For this review, take the finished solid that the model builds, in its own axes (mm). Face numbers are marked on the shaded views. A direction names the side the tool comes from. Round coordinates to 2 decimals unless told otherwise and drop trailing zeros. Loops run counter-clockwise (first coordinate to the right, second up) from the corner with the lowest first, then second, coordinate; pieces in that order, holes last.
1) Wall thickness on L1, parallel to Z at x = -84, y = -11; L2, parallel to Z at x = -97, y = -3.5; L3, parallel to Z at x = -57.5, y = 8: over which ranges is each line inside the solid? List them lowest first.
2) Take a section at A-A (x = -61). State the section outline as (y, z) points.
3) Take a section at C-C (z = -4). State the section outline as (x, y) points, then the cut area to 3 significant figures.
4) Insertion check: pin 1 (14.5 mm diameter, centred on x = -108.5, z = 19, fed in from +Y); pin 2 (11 mm diameter, centred on x = 27.5, z = -31.5, fed in from -Y); pin 3 (6.5 mm diameter, centred on y = -11, z = 17.06, fed in from +X); pin 4 (3 mm diameter, centred on x = 23.5, z = 16, fed in from -Y). Each pin has a flat end and moves straight along its axis. Give the tip position at first contact, or say it passes through.
5) Mouldability with a two-part tool opening along Z and no side actions: class the marked faces 4, 5 and 6 as pulls with the +Z half, pulls with the -Z half, needs draft (parallel to the pull), parting line crosses it, or undercut.
6) Take a section at B-B (x = 10). State the section outline as (y, z) points.
7) Tool access review of the marked faces 1, 2 and 3: name each direction out of +Z, -Z, +X, -X, +Y, -Y from which nothing blocks a thin tool from reaching the whole face with its end or side.
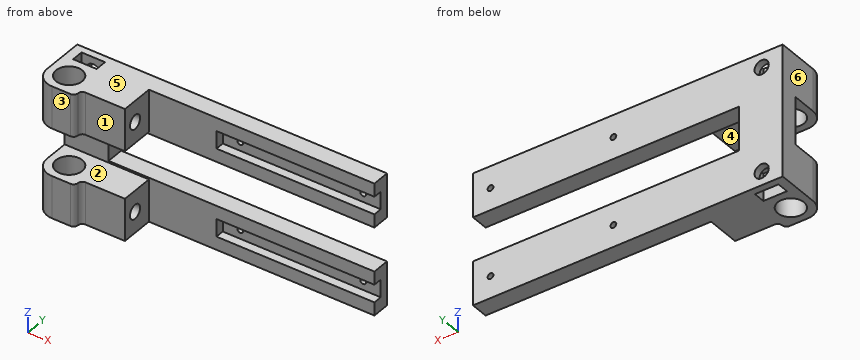
```python
from build123d import *

# Parameters (mm, degrees)
BOSS_EXTRUDE1_DEPTH = 10
SKETCH2_W           = 90
SKETCH2_H           = 10
CUT_EXTRUDE1_DEPTH  = 5
SKETCH3_R           = 1.65
CUT_EXTRUDE2_DEPTH  = 129.723786073
SKETCH5_W           = 23
SKETCH5_H           = 24
BOSS_EXTRUDE2_DEPTH = 24
SKETCH6_R           = 7.5
CUT_EXTRUDE3_DEPTH  = 144.649772109
SKETCH7_W           = 25
SKETCH7_H           = 24
BOSS_EXTRUDE3_DEPTH = 19
SKETCH8_R           = 4
CUT_EXTRUDE4_DEPTH  = 25
FILLET2_R           = 10
SKETCH12_W          = 13.4
SKETCH12_H          = 6.7
CUT_EXTRUDE5_DEPTH  = 15.5
CUT_EXTRUDE6_START  = -75
SKETCH12_2_W        = 13.4
SKETCH12_2_H        = 6.7
CUT_EXTRUDE6_DEPTH  = 15.5
CUT_EXTRUDE7_REACH  = 135.044
SKETCH13_R          = 4.05
FILLET3_R           = 2.5


with BuildPart() as part:
    # Sketch1 → Boss-Extrude1 (new body)
    with BuildSketch(Plane(origin=(0, 0, 0), x_dir=(1, 0, 0), z_dir=(0, 1, 0))):
        Polygon((-120.142652821, 45.940788785), (56.357347179, 45.940788785), (56.357347179, 20.940788785), (-95.142652821, 20.940788785), (-95.142652821, -4.059211215), (56.357347179, -4.059211215), (56.357347179, -29.059211215), (-120.142652821, -29.059211215), align=None)
    extrude(amount=BOSS_EXTRUDE1_DEPTH)

    # Sketch2 → Cut-Extrude1 (cut)
    with BuildSketch(Plane(origin=(0, 0, 0), x_dir=(1, 0, 0), z_dir=(0, 1, 0))):
        with Locations((11.357347179, 33.440788785)):
            Rectangle(SKETCH2_W, SKETCH2_H)
        with Locations((11.357347179, -16.559211215)):
            Rectangle(SKETCH2_W, SKETCH2_H)
    extrude(amount=CUT_EXTRUDE1_DEPTH, mode=Mode.SUBTRACT)

    # Sketch3 → Cut-Extrude2 (cut, through all)
    with BuildSketch(Plane(origin=(0, 5, 0), x_dir=(-1, 0, 0), z_dir=(0, -1, 0))):
        with Locations(Location((23.642652821, 33.440788785, 0), (0, 0, 90))):
            Circle(SKETCH3_R)
        with Locations(Location((-46.357347179, 33.440788785, 0), (0, 0, 90))):
            Circle(SKETCH3_R)
        with Locations(Location((23.642652821, -16.559211215, 0), (0, 0, 90))):
            Circle(SKETCH3_R)
        with Locations(Location((-46.357347179, -16.559211215, 0), (0, 0, 90))):
            Circle(SKETCH3_R)
    extrude(amount=-CUT_EXTRUDE2_DEPTH, mode=Mode.SUBTRACT)

    # Sketch5 → Boss-Extrude2 (add)
    with BuildSketch(Plane.XZ):
        with Locations((-108.642652821, 17.059211215)):
            Rectangle(SKETCH5_W, SKETCH5_H)
        with Locations((-108.642652821, -33.940788785)):
            Rectangle(SKETCH5_W, SKETCH5_H)
    extrude(amount=BOSS_EXTRUDE2_DEPTH)

    # Sketch6 → Cut-Extrude3 (cut, through all)
    with BuildSketch(Plane.XY.offset(29.059211215)):
        with Locations((-108.642652821, -12.5)):
            Circle(SKETCH6_R)
    extrude(amount=-CUT_EXTRUDE3_DEPTH, mode=Mode.SUBTRACT)

    # Sketch7 → Boss-Extrude3 (add)
    with BuildSketch(Plane.XZ):
        with Locations((-84.642652821, -33.940788785)):
            Rectangle(SKETCH7_W, SKETCH7_H)
        with Locations((-84.642652821, 17.059211215)):
            Rectangle(SKETCH7_W, SKETCH7_H)
    extrude(amount=BOSS_EXTRUDE3_DEPTH)

    # Sketch8 → Cut-Extrude4 (cut)
    with BuildSketch(Plane.ZY.offset(72.142652821)):
        with Locations(Location((-33.940788785, -11, 0), (0, 0, 180))):
            Circle(SKETCH8_R)
        with Locations(Location((17.059211215, -11, 0), (0, 0, 180))):
            Circle(SKETCH8_R)
    extrude(amount=CUT_EXTRUDE4_DEPTH, mode=Mode.SUBTRACT)

    # Fillet2
    fillet2_edges = [part.edges().sort_by_distance(p)[0] for p in [
        (-120.142652821, -24, 17.059211215),
        (-120.142652821, -24, -33.940788785),
    ]]
    fillet(fillet2_edges, radius=FILLET2_R)

    # Sketch12 → Cut-Extrude5 (cut)
    with BuildSketch(Plane(origin=(0, 0, -45.940788785), x_dir=(-1, 0, 0), z_dir=(0, 0, -1))):
        with Locations((108.142652821, 2.65)):
            Rectangle(SKETCH12_W, SKETCH12_H)
    extrude(amount=-CUT_EXTRUDE5_DEPTH, mode=Mode.SUBTRACT)

    # Sketch12<2> → Cut-Extrude6 (cut)
    with BuildSketch(Plane(origin=(0, 0, -45.940788785), x_dir=(-1, 0, 0), z_dir=(0, 0, -1)).offset(CUT_EXTRUDE6_START)):
        with Locations((108.142652821, 2.65)):
            Rectangle(SKETCH12_2_W, SKETCH12_2_H)
    extrude(amount=CUT_EXTRUDE6_DEPTH, mode=Mode.SUBTRACT)

    # Sketch13 → Cut-Extrude7 (cut, up to next)
    with BuildSketch(Plane(origin=(0, 10, 0), x_dir=(1, 0, 0), z_dir=(0, 1, 0)), mode=Mode.PRIVATE) as cut_extrude7_sk1:
        with Locations(Location((-108.142652821, 37.940788785, 0), (0, 0, 270))):
            Circle(SKETCH13_R)
    cut_extrude7_tool1 = extrude(cut_extrude7_sk1.sketch, amount=-CUT_EXTRUDE7_REACH, mode=Mode.PRIVATE) & part.part
    # Sketch13 → Cut-Extrude7 (cut, up to next)
    with BuildSketch(Plane(origin=(0, 10, 0), x_dir=(1, 0, 0), z_dir=(0, 1, 0)), mode=Mode.PRIVATE) as cut_extrude7_sk2:
        with Locations(Location((-108.142652821, -21.059211215, 0), (0, 0, 270))):
            Circle(SKETCH13_R)
    cut_extrude7_tool2 = extrude(cut_extrude7_sk2.sketch, amount=-CUT_EXTRUDE7_REACH, mode=Mode.PRIVATE) & part.part
    add(cut_extrude7_tool1.solids().sort_by_distance((-108.142653, 10, -37.940789))[0], mode=Mode.SUBTRACT)
    add(cut_extrude7_tool2.solids().sort_by_distance((-108.142653, 10, 21.059211))[0], mode=Mode.SUBTRACT)

    # Fillet3
    fillet3_edges = [part.edges().sort_by_distance(p)[0] for p in [
        (-97.142652821, -19, -33.940788785),
        (-97.142652821, -19, 17.059211215),
    ]]
    fillet(fillet3_edges, radius=FILLET3_R)
    fillet3_2_edges = [part.edges().sort_by_distance(p)[0] for p in [
        (-97.142652821, -24, -33.940788785),
        (-97.142652821, -24, 17.059211215),
    ]]
    fillet(fillet3_2_edges, radius=FILLET3_R - 0.0001)  # a hair under: the kernel refuses the full size


solid = part.part
```
Response:
1. L1: z = -45.94 to -37.94, -29.94 to -21.94, 5.06 to 13.06, 21.06 to 29.06
1. L2: z = -45.94 to -21.94, 5.06 to 29.06
1. L3: z = -45.94 to -20.94, 4.06 to 29.06
2. outline: (0, -45.94) - (10, -45.94) - (10, -20.94) - (0, -20.94) - close; (0, 4.06) - (10, 4.06) - (10, 29.06) - (0, 29.06) - close
3. outline: (-120.14, 0) - (-95.14, 0) - (-95.14, 10) - (-120.14, 10) - close
3. area: 250 mm2
4. pin 1: stops at y = 10
4. pin 2: stops at y = 0
4. pin 3: stops at x = -97.14
4. pin 4: stops at y = 5
5. face 4: undercut
5. face 5: pulls with the +Z half
5. face 6: needs draft
6. outline: (0, -45.94) - (10, -45.94) - (10, -20.94) - (0, -20.94) - (0, -28.44) - (5, -28.44) - (5, -38.44) - (0, -38.44) - close; (0, 4.06) - (10, 4.06) - (10, 29.06) - (0, 29.06) - (0, 21.56) - (5, 21.56) - (5, 11.56) - (0, 11.56) - close
7. face 1: +Z, -Z, +X, -Y
7. face 2: +X, -X, -Y
7. face 3: +Z, -Z, +X, -X, -Y
